Verification items for the finished model (mm, model axes). A direction names the side the tool comes from. Give positions to 0.01 mm unless a question says otherwise; leave off trailing zeros. Order: outer loops, then holes, each group sorted by start corner. A loop starts at its lowest first (then second) coordinate and runs counter-clockwise, first axis right, second up. Notation, with made-up numbers: (-1, 73.25) -> (6, 73.25) arc R31 cw to (6, 100.25) -> close; hole circle Ø7 at (45, -22). An arc over 180 degrees is marked (long way). Return JSON: item names as keys, results as strings. Group by question number.
(1) Cross-section at B-B on x = 24.5. Enter the section's corners in (y, z).
(2) Release check for a two-part mould opening along X. For faces 5 (the face through (20.93, 23.846, 7.509)), 6 (the face through (23.5, 5, -10)), 7 (the face through (16, -11, 17)) record: pulls with the +X half, pulls with the -X half, needs draft (parallel to the pull), parting line crosses it, or undercut.
(3) Cross-section at D-D on y = -19. Enter the section's corners in (x, z) (3 decimals), then the cut area to 3 significant figures.
(4) Tool access check on faces 1 (the face through (36, 0, 0)), 2 (the face through (9.12, -13.887, -10.648)), 3 (the face through (18.5, 12, -13)), 4 (the face through (30.93, 11.923, 3.755)). Record the directions out of +Z, -Z, +X, -X, +Y, -Y that give a thin tool (end or side, any length) a straight path to the whole face; none if there is none.
(5) Cross-section at A-A on y = 0. Enter the section's corners in (x, z).
(6) Thickness scan on line 1 along Z through (x, y) = (29.25, 0); line 2 along X through (y, z) = (20, 2); line 3 along Z through (x, y) = (22, 0). Record the ranges inside material, lowest first.
(7) Depth check by flat-ended pin: pin 1 Ø22.5 at (y, z) = (-5.5, 1.5) entering from -X; pin 2 Ø1 at (x, y) = (23, 7.5) entering from -Z; pin 3 Ø2 at (x, y) = (10.5, 13) entering from -Z; pin 4 Ø12 at (y, z) = (-10, -10) entering from +X. Enter the tip coordinate at first touch or a pass-through.
from build123d import *

# Parameters (mm, degrees)
F0_R     = 20
F1_DEPTH = 16
F2_R     = 25
F2_R_2   = 20
F3_DEPTH = 10
F4_R     = 12.5
F5_DEPTH = 10
F6_T     = -2.5


with BuildPart() as f1:
    # F0 (on Right) → F1 (new body)
    with BuildSketch(Plane.YZ):
        Circle(F0_R)
    extrude(amount=F1_DEPTH)

    # F2 (on face) → F3 (join)
    with BuildSketch(Plane.YZ.offset(16)):
        Circle(F2_R)
        Circle(F2_R_2, mode=Mode.SUBTRACT)
        Circle(F2_R_2)
    extrude(amount=F3_DEPTH)

    # F4 (on face) → F5 (join)
    with BuildSketch(Plane.YZ.offset(26)):
        Circle(F4_R)
    extrude(amount=F5_DEPTH)

    # F6
    f6_openings = [f1.faces().sort_by_distance(p)[0] for p in [
        (0, 0, 0),
    ]]
    offset(amount=F6_T, openings=f6_openings, kind=Kind.INTERSECTION)


solid = f1.part
Verdict:
{
 "1": {"outline": "circle Ø50 at (0, 0); hole circle Ø20 at (0, 0)"},
 "2": {"face 5": "needs draft", "face 6": "undercut", "face 7": "pulls with the -X half"},
 "3": {"outline": "(0, -6.245) -> (16, -6.245) -> (16, -16.248) -> (26, -16.248) -> (26, 16.248) -> (16, 16.248) -> (16, 6.245) -> (0, 6.245) -> close; hole (18.5, -12.052) -> (23.5, -12.052) -> (23.5, 12.052) -> (18.5, 12.052) -> close", "area": "404 mm²"},
 "4": {"face 1": "+Z, -Z, +X, +Y, -Y", "face 2": "-X", "face 3": "none", "face 4": "+X"},
 "5": {"outline": "(0, -20) -> (16, -20) -> (16, -25) -> (26, -25) -> (26, -12.5) -> (36, -12.5) -> (36, 12.5) -> (26, 12.5) -> (26, 25) -> (16, 25) -> (16, 20) -> (0, 20) -> (0, 17.5) -> (18.5, 17.5) -> (18.5, 22.5) -> (23.5, 22.5) -> (23.5, 10) -> (33.5, 10) -> (33.5, -10) -> (23.5, -10) -> (23.5, -22.5) -> (18.5, -22.5) -> (18.5, -17.5) -> (0, -17.5) -> close"},
 "6": {"line 1": "-12.5 to -10, 10 to 12.5", "line 2": "16 to 18.5, 23.5 to 26", "line 3": "-25 to -22.5, 22.5 to 25"},
 "7": {"pin 1": "x = 23.5", "pin 2": "z = -24", "pin 3": "z = -16", "pin 4": "x = 36"}
}
